Model file for the job. Use its own axes, mm. Face numbers are marked on the shaded views. A direction names the side the tool comes from. Give positions to 0.01 mm unless a question says otherwise; leave off trailing zeros. Write each loop counter-clockwise with the first axis right and the second up, starting at its lowest first coordinate (ties: lowest second). Pieces come first, ordered by that corner, then holes. Notation, with made-up numbers: (-25, -14) - (6, -14) arc R27 cw to (6, 15) - close; hole circle Ø9 at (68.5, 59). An arc over 180 degrees is marked (long way). One line per item, written item: value. Start each with the question number.
(1) Probe L1, parallel to Y at x = 0, z = 1.25; L2, parallel to X at y = -11.5, z = 0; L3, parallel to Y at x = 0, z = -6.5. List the from-to ranges inside material, lowest first.
(2) 3-axis set-ups, long thin cutter, end or side, ignore diameter. For the marked faces 4, 5 and 6: which of +Z, -Z, +X, -X, +Y, -Y reach the whole face in a straight line?
(3) Cut at D-D, the plane z = 7. List the corners of the cut face in (x, y), and give its area (3 significant figures).
(4) Cut at C-C, the plane y = -3. List the corners of the cut face in (x, z), and give its area (3 significant figures).
(5) Cut at A-A, the plane x = 0. List the corners of the cut face in (y, z), and give its area (3 significant figures).
(6) Cut at B-B, the plane z = 0. List the corners of the cut face in (x, y).
(7) Drop flat-ended pins along their axis: P1, Ø3, axis at y = 4, z = -5.5, coming from the +X side; P2, Ø8, axis at x = -2.5, y = -1.5, coming from the +Z side; P3, Ø1.5, axis at x = -5, y = -2.5, coming from the -Z side. Give the stop position or say it passes through.
(8) Mould opens along Z. For the marked faces 1, 2 and 3 say: pulls with the +Z half, pulls with the -Z half, needs draft (parallel to the pull), parting line crosses it, or undercut.
from build123d import *

# Parameters (mm, degrees)
BOSS_EXTRUDE2_DEPTH = 9.5
SKETCH4_R           = 4
CUT_EXTRUDE1_DEPTH  = 27.097174177
SKETCH9_R           = 8.1
CUT_EXTRUDE3_DEPTH  = 5
CUT_EXTRUDE4_START  = -5
SKETCH10_R          = 8.1
CUT_EXTRUDE4_DEPTH  = 5
SKETCH12_R          = 2.55
CUT_EXTRUDE6_DEPTH  = 8
FILLET1_R           = 0.5


with BuildPart() as part:
    # Sketch3 → Boss-Extrude2 (new, symmetric)
    with BuildSketch(Plane.XY):
        with BuildLine():
            Line((9.75, 0), (9.75, -15))
            Line((9.75, -15), (-9.75, -15))
            Line((-9.75, -15), (-9.75, 0))
            ThreePointArc((-9.75, 0), (0, 9.75), (9.75, 0))
        make_face()
    extrude(amount=BOSS_EXTRUDE2_DEPTH, both=True)

    # Sketch4 → Cut-Extrude1 (cut, through all)
    with BuildSketch(Plane(origin=(0, 0, -9.5), x_dir=(-1, 0, 0), z_dir=(0, 0, -1))):
        Circle(SKETCH4_R)
    extrude(amount=-CUT_EXTRUDE1_DEPTH, mode=Mode.SUBTRACT)

    # Sketch9 → Cut-Extrude3 (cut)
    with BuildSketch(Plane(origin=(0, 0, -9.5), x_dir=(-1, 0, 0), z_dir=(0, 0, -1))):
        Circle(SKETCH9_R)
    extrude(amount=-CUT_EXTRUDE3_DEPTH, mode=Mode.SUBTRACT)

    # Sketch10 → Cut-Extrude4 (cut)
    with BuildSketch(Plane.XY.offset(9.5).offset(CUT_EXTRUDE4_START)):
        with Locations(Location((0, 0, 0), (0, 0, 180))):
            Circle(SKETCH10_R)
    extrude(amount=CUT_EXTRUDE4_DEPTH, mode=Mode.SUBTRACT)

    # Sketch12 → Cut-Extrude6 (cut)
    with BuildSketch(Plane.XZ.offset(15)):
        with Locations(Location((0, 0, 0), (0, 0, 270))):
            Circle(SKETCH12_R)
    extrude(amount=-CUT_EXTRUDE6_DEPTH, mode=Mode.SUBTRACT)

    # Fillet1
    fillet1_edges = [part.edges().sort_by_distance(p)[0] for p in [
        (9.75, -7.5, 9.5),
        (0, 9.75, 9.5),
        (9.75, -7.5, -9.5),
        (-9.75, -7.5, -9.5),
        (0, 9.75, -9.5),
        (-9.75, -7.5, 9.5),
    ]]
    fillet(fillet1_edges, radius=FILLET1_R)


solid = part.part
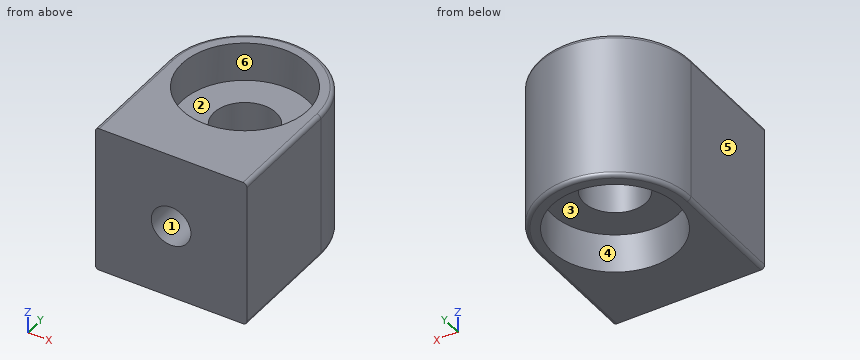
Answers follow:
1. L1: y = -7 to -4, 4 to 9.75
1. L2: x = -9.75 to -2.55, 2.55 to 9.75
1. L3: y = -15 to -8.1, 8.1 to 9.75
2. face 4: -Z
2. face 5: +Z, -Z, -X, +Y, -Y
2. face 6: +Z
3. outline: (-9.75, -15) - (9.75, -15) - (9.75, 0) arc R9.75 ccw to (-9.75, 0) - close; hole circle Ø16.2 at (0, 0)
3. area: 236 mm²
4. outline: (-9.75, -9) arc R0.5 ccw to (-9.25, -9.5) - (-7.52, -9.5) - (-7.52, -4.5) - (-2.65, -4.5) - (-2.65, 4.5) - (-7.52, 4.5) - (-7.52, 9.5) - (-9.25, 9.5) arc R0.5 ccw to (-9.75, 9) - close; (2.65, -4.5) - (7.52, -4.5) - (7.52, -9.5) - (9.25, -9.5) arc R0.5 ccw to (9.75, -9) - (9.75, 9) arc R0.5 ccw to (9.25, 9.5) - (7.52, 9.5) - (7.52, 4.5) - (2.65, 4.5) - close
4. area: 172 mm²
5. outline: (-15, -9.5) - (-8.1, -9.5) - (-8.1, -4.5) - (-4, -4.5) - (-4, 4.5) - (-8.1, 4.5) - (-8.1, 9.5) - (-15, 9.5) - (-15, 2.55) - (-7, 2.55) - (-7, -2.55) - (-15, -2.55) - close; (4, -4.5) - (8.1, -4.5) - (8.1, -9.5) - (9.25, -9.5) arc R0.5 ccw to (9.75, -9) - (9.75, 9) arc R0.5 ccw to (9.25, 9.5) - (8.1, 9.5) - (8.1, 4.5) - (4, 4.5) - close
5. area: 195 mm²
6. outline: (-9.75, -15) - (-2.55, -15) - (-2.55, -7) - (2.55, -7) - (2.55, -15) - (9.75, -15) - (9.75, 0) arc R9.75 ccw to (-9.75, 0) - close; hole circle Ø8 at (0, 0)
7. P1: stops at x = 9.42
7. P2: stops at z = 4.5
7. P3: stops at z = -4.5
8. face 1: undercut
8. face 2: pulls with the +Z half
8. face 3: pulls with the -Z half
